from build123d import *

# Parameters (mm, degrees)
SKETCH1_R           = 15
SKETCH1_R_2         = 13
BOSS_EXTRUDE1_DEPTH = 10
SKETCH1_2_R         = 15
SKETCH1_2_R_2       = 13
BOSS_EXTRUDE2_DEPTH = 10
BOSS_EXTRUDE3_START = 2
SKETCH2_R           = 15
BOSS_EXTRUDE3_DEPTH = 2
SKETCH3_W           = 21.803591486
SKETCH3_H           = 3.802953439
BOSS_EXTRUDE4_DEPTH = 20
FILLET1_R           = 8
CUT_EXTRUDE1_REACH  = 38.732
SKETCH4_R           = 5


with BuildPart() as part:
    # Sketch1 → Boss-Extrude1 (new body)
    with BuildSketch(Plane.XY):
        Circle(SKETCH1_R)
        Circle(SKETCH1_R_2, mode=Mode.SUBTRACT)
    extrude(amount=BOSS_EXTRUDE1_DEPTH)

    # Sketch1<2> → Boss-Extrude2 (add)
    with BuildSketch(Plane.XY):
        Circle(SKETCH1_2_R)
        Circle(SKETCH1_2_R_2, mode=Mode.SUBTRACT)
    extrude(amount=BOSS_EXTRUDE2_DEPTH)

    # Sketch2 → Boss-Extrude3 (add)
    with BuildSketch(Plane(origin=(0, 0, 0), x_dir=(-1, 0, 0), z_dir=(0, 0, -1)).offset(BOSS_EXTRUDE3_START)):
        Circle(SKETCH2_R)
    extrude(amount=-BOSS_EXTRUDE3_DEPTH)

    # Sketch3 → Boss-Extrude4 (add)
    with BuildSketch(Plane(origin=(0, 0, -2), x_dir=(-1, 0, 0), z_dir=(0, 0, -1))):
        with Locations((0, -8.401476719)):
            Rectangle(SKETCH3_W, SKETCH3_H)
        with Locations((0, 8.401476719)):
            Rectangle(SKETCH3_W, SKETCH3_H)
    extrude(amount=BOSS_EXTRUDE4_DEPTH)

    # Fillet1
    fillet1_edges = [part.edges().sort_by_distance(p)[0] for p in [
        (-10.901795743, -8.40147672, -22),
        (10.901795743, -8.40147672, -22),
        (10.901795743, 8.40147672, -22),
        (-10.901795743, 8.40147672, -22),
    ]]
    fillet(fillet1_edges, radius=FILLET1_R)

    # Cut-Extrude1: up to this face of the body (flat: up to its plane)
    cut_extrude1_end = Plane(part.part.faces().sort_by_distance((0, -10.302953439, -11.447862962))[0])
    # Sketch4 → Cut-Extrude1 (cut, up to the picked face)
    with BuildSketch(Plane(origin=(0, 10.302953439, 0), x_dir=(1, 0, 0), z_dir=(0, 1, 0)), mode=Mode.PRIVATE) as cut_extrude1_sk1:
        with Locations(Location((0, 14, 0), (0, 0, 270))):
            Circle(SKETCH4_R)
    cut_extrude1_tool1 = split(extrude(cut_extrude1_sk1.sketch, amount=-CUT_EXTRUDE1_REACH, mode=Mode.PRIVATE), bisect_by=cut_extrude1_end, keep=Keep.BOTH, mode=Mode.PRIVATE)
    add(cut_extrude1_tool1.solids().sort_by(Axis((0, 10.302953, -14), (0, -1, 0)))[0], mode=Mode.SUBTRACT)


solid = part.part
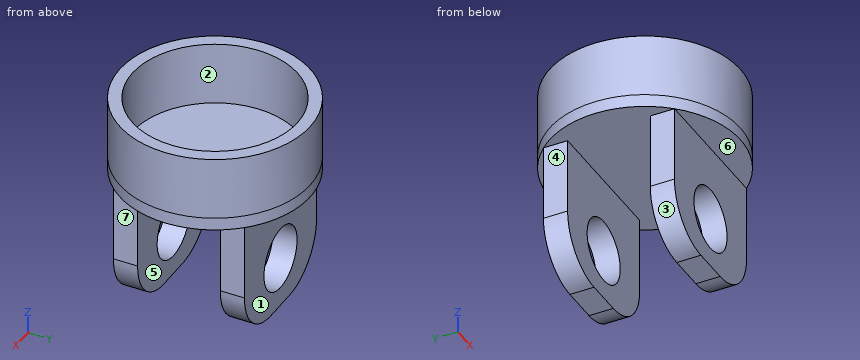
For this review, take the finished solid that the model builds, in its own axes (mm). Face numbers are marked on the shaded views. A direction names the side the tool comes from. Round coordinates to 2 decimals unless told otherwise and drop trailing zeros. Write each loop counter-clockwise with the first axis right and the second up, starting at its lowest first coordinate (ties: lowest second). Pieces come first, ordered by that corner, then holes. Notation, with made-up numbers: (12.25, 42) -> (42.25, 42) arc R17 ccw to (42.25, 68) -> close; hole circle Ø6 at (5, 46.25). An arc over 180 degrees is marked (long way). Put each result on its own line as item: value.
Q1. Consider section D-D on y = 0. State the section outline as (x, z) points, and give its area (3 significant figures).
Determined:
outline: (-15, -2) -> (15, -2) -> (15, 10) -> (13, 10) -> (13, 0) -> (-13, 0) -> (-13, 10) -> (-15, 10) -> close
area: 100 mm^2
Q2. Consider section A-A on x = 0. State the section outline as (y, z) points.
Determined:
outline: (-15, -2) -> (-10.3, -2) -> (-10.3, -9) -> (-6.5, -9) -> (-6.5, -2) -> (6.5, -2) -> (6.5, -9) -> (10.3, -9) -> (10.3, -2) -> (15, -2) -> (15, 10) -> (13, 10) -> (13, 0) -> (-13, 0) -> (-13, 10) -> (-15, 10) -> close; (-10.3, -22) -> (-6.5, -22) -> (-6.5, -19) -> (-10.3, -19) -> close; (6.5, -22) -> (10.3, -22) -> (10.3, -19) -> (6.5, -19) -> close
Q3. Consider section C-C on z = -3.5. State the section outline as (x, y) points.
Determined:
outline: (-10.9, -10.3) -> (10.9, -10.3) -> (10.9, -6.5) -> (-10.9, -6.5) -> close; (-10.9, 6.5) -> (10.9, 6.5) -> (10.9, 10.3) -> (-10.9, 10.3) -> close
Q4. Machinability: for the marked faces 4, 5, 6 and 7, which of the approach directions +Z, -Z, +X, -X, +Y, -Y give a long, thin tool a straight path to every point of the face, cutting with its end or side? Answer none if there is none.
Determined:
face 4: -Z, -X, +Y, -Y
face 5: -Z, +X, -X
face 6: -Z, +X, -X, -Y
face 7: -Z, +X, +Y, -Y
Q5. Clearance check with flat-ended pins moving along their axes: pin 1 Ø3 at (x, z) = (10.5, 6) entering from +Y; pin 2 Ø2.5 at (x, y) = (4, 13.5) entering from -Z; pin 3 Ø2 at (x, y) = (-3, -2) entering from +Z. State where each tip first meets the part, or that it passes through.
Determined:
pin 1: stops at y = 12
pin 2: stops at z = -2
pin 3: stops at z = 0
Q6. The part is to be moulded in two halves that separate along Y. For the marked faces 1, 2 and 3, say which applies: released by +Y, released by -Y, zero draft, split by the parting line, or undercut.
Determined:
face 1: released by +Y
face 2: undercut
face 3: zero draft
Q7. Consider section B-B on z = -18. State the section outline as (x, y) points.
Determined:
outline: (-9.83, -10.3) -> (-3, -10.3) -> (-3, -6.5) -> (-9.83, -6.5) -> close; (-9.83, 6.5) -> (-3, 6.5) -> (-3, 10.3) -> (-9.83, 10.3) -> close; (3, -10.3) -> (9.83, -10.3) -> (9.83, -6.5) -> (3, -6.5) -> close; (3, 6.5) -> (9.83, 6.5) -> (9.83, 10.3) -> (3, 10.3) -> close
Q8. To check wall thickness, follow L1, parallel to X at y = 7.7, z = -14; L2, parallel to Y at x = 5.75, z = -17.5; L3, parallel to Y at x = 0, z = 7.25. State the ranges of each line that lie inside material, in increasing order. Write a range as [from, to].
Determined:
L1: x = [-10.9, -5], [5, 10.9]
L2: y = [-10.3, -6.5], [6.5, 10.3]
L3: y = [-15, -13], [13, 15]
